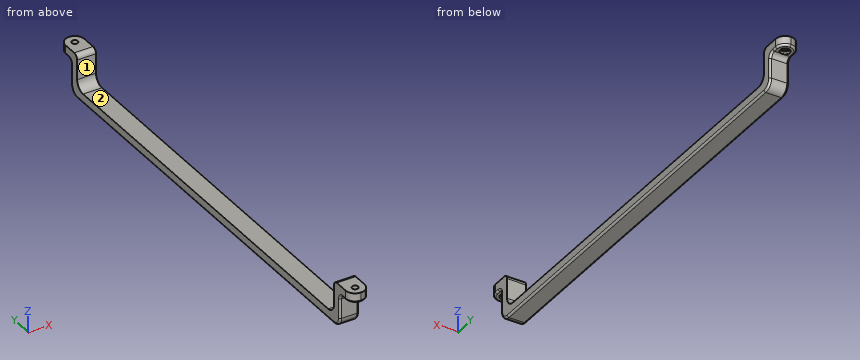
```python
from build123d import *

# Parameters (mm, degrees)
BOSS_EXTRUDE1_DEPTH = 5
BOSS_EXTRUDE2_DEPTH = 18
SKETCH3_W           = 9.999999999999972
SKETCH3_H           = 10
BOSS_EXTRUDE3_DEPTH = 5
SKETCH4_R           = 1.5999999999999999
SKETCH4_R_2         = 1.599999999999992
CUT_EXTRUDE1_DEPTH  = 241.88171371027735
SKETCH5_R           = 2.5000000000000004
SKETCH5_R_2         = 2.500000000000001
CUT_EXTRUDE2_DEPTH  = 1.5
FILLET1_R           = 5
FILLET2_R           = 2.5
FILLET3_R           = 1


with BuildPart() as part:
    # Sketch1 → Boss-Extrude1 (new body)
    with BuildSketch(Plane.XY):
        Polygon((0, 0), (0, 230), (9.999999999999972, 230), (10, -7.8e-16), align=None)
    extrude(amount=BOSS_EXTRUDE1_DEPTH)

    # Sketch2 → Boss-Extrude2 (add)
    with BuildSketch(Plane.XY.offset(5)):
        Polygon((0, 0), (10, -7.8e-16), (10, 4.999999999999999), (0, 5.000000000000004), align=None)
        Polygon((0, 230), (9.999999999999972, 230), (10, 225), (0, 225), align=None)
    extrude(amount=BOSS_EXTRUDE2_DEPTH)

    # Sketch3 → Boss-Extrude3 (add)
    with BuildSketch(Plane.XY.offset(23)):
        with Locations((4.999999999999986, 235.00000000000003)):
            Rectangle(SKETCH3_W, SKETCH3_H)
        Polygon((0, 0), (10, -7.8e-16), (10.000000000000002, -10), (0, -10.000000000000002), align=None)
    extrude(amount=-BOSS_EXTRUDE3_DEPTH)

    # Sketch4 → Cut-Extrude1 (cut, through all)
    with BuildSketch(Plane(origin=(0, 0, 18), x_dir=(-1, 0, 0), z_dir=(0, 0, -1))):
        with Locations((-5, -5.000000000000002)):
            Circle(SKETCH4_R)
        with Locations((-5, 235.00000000000003)):
            Circle(SKETCH4_R_2)
    extrude(amount=-CUT_EXTRUDE1_DEPTH, mode=Mode.SUBTRACT)

    # Sketch5 → Cut-Extrude2 (cut)
    with BuildSketch(Plane(origin=(0, 0, 18), x_dir=(-1, 0, 0), z_dir=(0, 0, -1))):
        with Locations((-5, -5.000000000000002)):
            Circle(SKETCH5_R)
        with Locations((-5, 235.00000000000003)):
            Circle(SKETCH5_R_2)
    extrude(amount=-CUT_EXTRUDE2_DEPTH, mode=Mode.SUBTRACT)

    # Fillet1
    fillet1_edges = [part.edges().sort_by_distance(p)[0] for p in [
        (0, -10.000000000000002, 20.5),
        (10.000000000000002, -10, 20.5),
        (0, 240.00000000000003, 20.5),
        (9.999999999999972, 240.00000000000003, 20.5),
        (5, 225, 5),
        (4.999999999999986, 230, 0),
        (5, 5.000000000000002, 5),
        (5, -3.9e-16, 0),
    ]]
    fillet(fillet1_edges, radius=FILLET1_R - 0.0001)  # a hair under: the kernel refuses the full size

    # Fillet2
    fillet2_edges = [part.edges().sort_by_distance(p)[0] for p in [
        (5, 5.000000000000002, 23),
        (5, 225, 23),
        (4.999999999999986, 230, 18),
        (5, -3.9e-16, 18),
    ]]
    fillet(fillet2_edges, radius=FILLET2_R)

    # Fillet3
    fillet3_edges = [part.edges().sort_by_distance(p)[0] for p in [
        (0, 115, 0),
        (0, 233.75005000000002, 18),
        (-2.7e-16, 1.4644368047453802, 1.4644368047453806),
        (0, 228.5355631952546, 1.4644368047453806),
        (10, -3.7500500000000008, 18),
        (8.53556319525462, -8.535563195254621, 18),
        (1.464436804745381, -8.53556319525462, 18),
        (9.999999999999986, 115, 0),
        (10, 1.4644368047453793, 1.4644368047453806),
        (9.999999999999972, 228.5355631952546, 1.4644368047453806),
        (8.53556319525459, 238.53556319525464, 18),
        (1.4644368047453793, 238.53556319525464, 18),
        (10, -7.8e-16, 10.249949999999998),
        (9.999999999999972, 230, 10.24995),
        (9.999999999999972, 233.75005000000002, 18),
        (0, -3.75005, 18),
        (0, 230, 10.24995),
        (0, 0, 10.249949999999998),
        (9.999999999999972, 230.73223304703362, 17.26776695296637),
        (0, 230.73223304703362, 17.26776695296637),
        (1.4e-16, -0.7322330470336309, 17.26776695296637),
        (10, -0.7322330470336316, 17.26776695296637),
    ]]
    fillet(fillet3_edges, radius=FILLET3_R)


solid = part.part
```
Geometry check sheet. Reference: the model listing, model coordinates, mm. Face numbers are marked on the shaded views. Round coordinates to 2 decimals unless told otherwise and drop trailing zeros. Loops run counter-clockwise (first coordinate to the right, second up) from the corner with the lowest first, then second, coordinate; pieces in that order, holes last. Notation, with made-up numbers: (24.5, -40) - (33.5, -40) arc R23 cw to (33.5, -21) - close; hole circle Ø5 at (32.5, -33.75). An arc over 180 degrees is marked (long way). Write item = value, one per line. Start each with the question number.
1. Depth check by flat-ended pin: pin 1 (6 mm diameter, centred on x = 5, y = 106.5, fed in from +Z); pin 2 (5.5 mm diameter, centred on x = 5, y = 236, fed in from -Z); pin 3 (2.5 mm diameter, centred on x = 6.5, z = 11, fed in from -Y); pin 4 (6 mm diameter, centred on x = 5, y = -5, fed in from +Z). Enter the tip coordinate at first touch or a pass-through.
2. Thickness scan on line 1 (Y direction, x = 2.25, z = 10.75); line 2 (Y direction, x = 7, z = 18.5); line 3 (Z direction, x = 4, y = 168). Record the ranges inside material, lowest first.
3. Mould release check, pull along Y, two halves, no side actions. Record for the marked faces 1 and 2: released by +Y, released by -Y, zero draft, split by the parting line, or undercut.
4. Section check A-A on y = 133.5. Enter the section's corners in (x, z), then the cut area to 3 significant figures.
Working result:
q1.pin_1 = 5
q1.pin_2 = 18
q1.pin_3 = 0
q1.pin_4 = 23
q2.line_1 = 0 to 5, 225 to 230
q2.line_2 = -9.44 to -6.5, -3.5 to 5, 225 to 233.5, 236.5 to 239.44
q2.line_3 = 0 to 5
q3.face_1 = undercut
q3.face_2 = undercut
q4.outline = (0, 1) arc R1 ccw to (1, 0) - (9, 0) arc R1 ccw to (10, 1) - (10, 5) - (0, 5) - close
q4.area = 49.6 mm^2
